```python
from build123d import *

# Parameters (mm, degrees)
F0_W     = 75
F0_H     = 12.5
F2_DEPTH = 3
F3_DEPTH = 25.4
F1_W     = 30.3805638105
F1_H     = 1.609168168
F1_H_2   = 8.2122374663
F1_H_3   = 1.5025624558
F1_H_4   = 8.1500614509
F4_DEPTH = 0.1
F5_R     = 2.54


# Not quite as in the source:
# - a feature names something its author has since deleted; it is built from what else it names


with BuildPart() as f2:
    # F0 (on Top) → F2 (new body)
    with BuildSketch(Plane.XY):
        with Locations((2.6580473056, -0.5825519562)):
            Rectangle(F0_W, F0_H)
        with Locations((2.6580473056, 11.9174480438)):
            Rectangle(F0_W, F0_H)
    extrude(amount=F2_DEPTH)

    # F1 (on face) → F3 (cut)
    with BuildSketch(Plane.XY):
        with BuildLine():
            ThreePointArc((37.4252376516, 5.6674480438), (37.4269210618, 5.709628552), (37.4274823308, 5.7518389076))
            ThreePointArc((37.4274823308, 5.7518389076), (36.7935957485, 7.0210030812), (35.3981560952, 7.2766162118))
            Line((35.3981560952, 7.2766162118), (35.8816406012, 7.2766162118))
            Line((35.8816406012, 7.2766162118), (35.8816406012, 5.6674480438))
            Line((35.8816406012, 5.6674480438), (37.4252376516, 5.6674480438))
        make_face()
        with BuildLine():
            Line((35.8816406012, 7.2766162118), (35.3981560952, 7.2766162118))
            ThreePointArc((35.3981560952, 7.2766162118), (34.5459110587, 6.6713691097), (34.25472701, 5.6674480438))
            Line((34.25472701, 5.6674480438), (35.8816406012, 5.6674480438))
            Line((35.8816406012, 5.6674480438), (35.8816406012, 7.2766162118))
        make_face()
        with BuildLine():
            ThreePointArc((35.8816406012, 4.164885588), (36.9472923333, 4.6142885534), (37.4252376516, 5.6674480438))
            Line((37.4252376516, 5.6674480438), (35.8816406012, 5.6674480438))
            Line((35.8816406012, 5.6674480438), (35.8816406012, 4.164885588))
        make_face()
        with BuildLine():
            Line((35.8816406012, 5.6674480438), (34.25472701, 5.6674480438))
            ThreePointArc((34.25472701, 5.6674480438), (34.7326723283, 4.6142885534), (35.7983240604, 4.164885588))
            Line((35.7983240604, 4.164885588), (35.8816406012, 4.164885588))
            Line((35.8816406012, 4.164885588), (35.8816406012, 5.6674480438))
        make_face()
        with BuildLine():
            Line((-30.5555813976, 5.6674480438), (-30.5555813976, 7.2766162118))
            ThreePointArc((-30.5555813976, 7.2766162118), (-31.6926900402, 6.8077826631), (-32.1536216159, 5.6674480438))
            Line((-32.1536216159, 5.6674480438), (-30.5555813976, 5.6674480438))
        make_face()
        with BuildLine():
            ThreePointArc((-28.9787699914, 5.6891521952), (-29.4399653273, 6.8078988393), (-30.5555813976, 7.2766162118))
            Line((-30.5555813976, 7.2766162118), (-30.5555813976, 5.6674480438))
            Line((-30.5555813976, 5.6674480438), (-28.9789183669, 5.6674480438))
            ThreePointArc((-28.9789183669, 5.6674480438), (-28.9788070858, 5.678299866), (-28.9787699914, 5.6891521952))
        make_face()
        with BuildLine():
            ThreePointArc((-30.1226850953, 4.164885588), (-29.303099666, 4.7276133355), (-28.9789183669, 5.6674480438))
            Line((-28.9789183669, 5.6674480438), (-30.5555813976, 5.6674480438))
            Line((-30.5555813976, 5.6674480438), (-30.5555813976, 4.164885588))
            Line((-30.5555813976, 4.164885588), (-30.1226850953, 4.164885588))
        make_face()
        with BuildLine():
            Line((-30.5555813976, 5.6674480438), (-32.1536216159, 5.6674480438))
            ThreePointArc((-32.1536216159, 5.6674480438), (-31.5104490346, 4.4129538625), (-30.1226850953, 4.164885588))
            Line((-30.1226850953, 4.164885588), (-30.5555813976, 4.164885588))
            Line((-30.5555813976, 4.164885588), (-30.5555813976, 5.6674480438))
        make_face()
    extrude(amount=F3_DEPTH, mode=Mode.SUBTRACT)

    # F1 (on face) → F4 (cut)
    with BuildSketch(Plane.XY):
        with BuildLine():
            ThreePointArc((34.25472701, 5.6674480438), (34.5459110587, 6.6713691097), (35.3981560952, 7.2766162118))
            Line((35.3981560952, 7.2766162118), (15.1902819052, 7.2766162118))
            Line((15.1902819052, 7.2766162118), (15.1902819052, 5.6674480438))
            Line((15.1902819052, 5.6674480438), (34.25472701, 5.6674480438))
        make_face()
        with BuildLine():
            ThreePointArc((35.7983240604, 4.164885588), (34.7326723283, 4.6142885534), (34.25472701, 5.6674480438))
            Line((34.25472701, 5.6674480438), (15.1902819052, 5.6674480438))
            Line((15.1902819052, 5.6674480438), (15.1902819052, 4.164885588))
            Line((15.1902819052, 4.164885588), (35.7983240604, 4.164885588))
        make_face()
        with Locations((0, 6.4720321278)):
            Rectangle(F1_W, F1_H)
        with Locations((0, 11.382734945)):
            Rectangle(F1_W, F1_H_2)
        with Locations((0, 4.9161668159)):
            Rectangle(F1_W, F1_H_3)
        with BuildLine():
            Line((-15.1902819052, 5.6674480438), (-15.1902819052, 7.2766162118))
            Line((-15.1902819052, 7.2766162118), (-30.5555813976, 7.2766162118))
            ThreePointArc((-30.5555813976, 7.2766162118), (-29.4399653273, 6.8078988393), (-28.9787699914, 5.6891521952))
            ThreePointArc((-28.9787699914, 5.6891521952), (-28.9788070858, 5.678299866), (-28.9789183669, 5.6674480438))
            Line((-28.9789183669, 5.6674480438), (-15.1902819052, 5.6674480438))
        make_face()
        with Locations((0, 0.0898548626)):
            Rectangle(F1_W, F1_H_4)
        with BuildLine():
            Line((-15.1902819052, 4.164885588), (-15.1902819052, 5.6674480438))
            Line((-15.1902819052, 5.6674480438), (-28.9789183669, 5.6674480438))
            ThreePointArc((-28.9789183669, 5.6674480438), (-29.303099666, 4.7276133355), (-30.1226850953, 4.164885588))
            Line((-30.1226850953, 4.164885588), (-15.1902819052, 4.164885588))
        make_face()
    extrude(amount=F4_DEPTH, mode=Mode.SUBTRACT)

    # F5
    f5_edges = [f2.edges().sort_by_distance(p)[0] for p in [
        (-15.190282, 4.164886, 0.05),
        (-15.190282, 7.276616, 0.05),
        (15.190282, 4.164886, 0.05),
        (15.190282, 7.276616, 0.05),
    ]]
    fillet(f5_edges, radius=F5_R)


solid = f2.part
```
Check sheet for the modelled part. Datum: model origin and axes. Units: mm. Coordinates: 2 decimals unless noted, no trailing zeros. Order: outer loops, then holes, each group sorted by start corner. A loop starts at its lowest first (then second) coordinate and runs counter-clockwise, first axis right, second up. Notation, with made-up numbers: (53, 35) -> (65, 35) arc R27 cw to (65, 57) -> close; hole circle Ø11 at (27.25, -24.75). An arc over 180 degrees is marked (long way). Write item = value, one per line. Start each with the question number.
1) Material ranges on L1, parallel to X at y = 5.75, z = 2.8; L2, parallel to X at y = 7, z = 1.75; L3, parallel to Z at x = -20, y = 5.25, recorded low to high.
2) Go/stop test with a flat-tipped pin: P1, Ø1, axis at x = -1, y = 14, coming from the -Z side. Record where the tip stops, or that it passes through.
3) Cross-section at A-A (x = 14.5). Enter the section's corners in (y, z).
4) Mould release check, pull along X, two halves, no side actions. Record for faces 1 (the flat face through (2, -5, 0)), 2 (the flat face through (2, 6, 0.1)), 3 (the flat face through (40.158, 5, 1)): +X half, -X half, draft (parallel to the pull), parting line (faces both ways), or undercut.
Ans:
q1.L1 = -34.84 to -32.15, -28.98 to 34.25, 37.43 to 40.16
q1.L2 = -34.84 to -31.46, -29.67 to 34.86, 36.82 to 40.16
q1.L3 = 0.1 to 3
q2.P1 = 0.1
q3.outline = (-6.83, 0) -> (-3.99, 0) -> (-3.99, 0.1) -> (15.49, 0.1) -> (15.49, 0) -> (18.17, 0) -> (18.17, 3) -> (-6.83, 3) -> close
q4.face_1 = draft
q4.face_2 = undercut
q4.face_3 = +X half
